Can you work these out from the drawing? Everything is in mm from the part's minimum corner. A direction names the side the tool comes from. Round coordinates to 2 decimals unless told otherwise and drop trailing zeros. Order: outer loops, then holes, each group sorted by start corner. A loop starts at its lowest first (then second) coordinate and runs counter-clockwise, first axis right, second up. Notation, with made-up numbers: M -2,78 L 54,78 A25 ccw 54,100 Z; hole C 1,81.5 d9. An arc over 180 degrees is marked long. Answer as a JSON object with one key per item and string values. Group by question number.
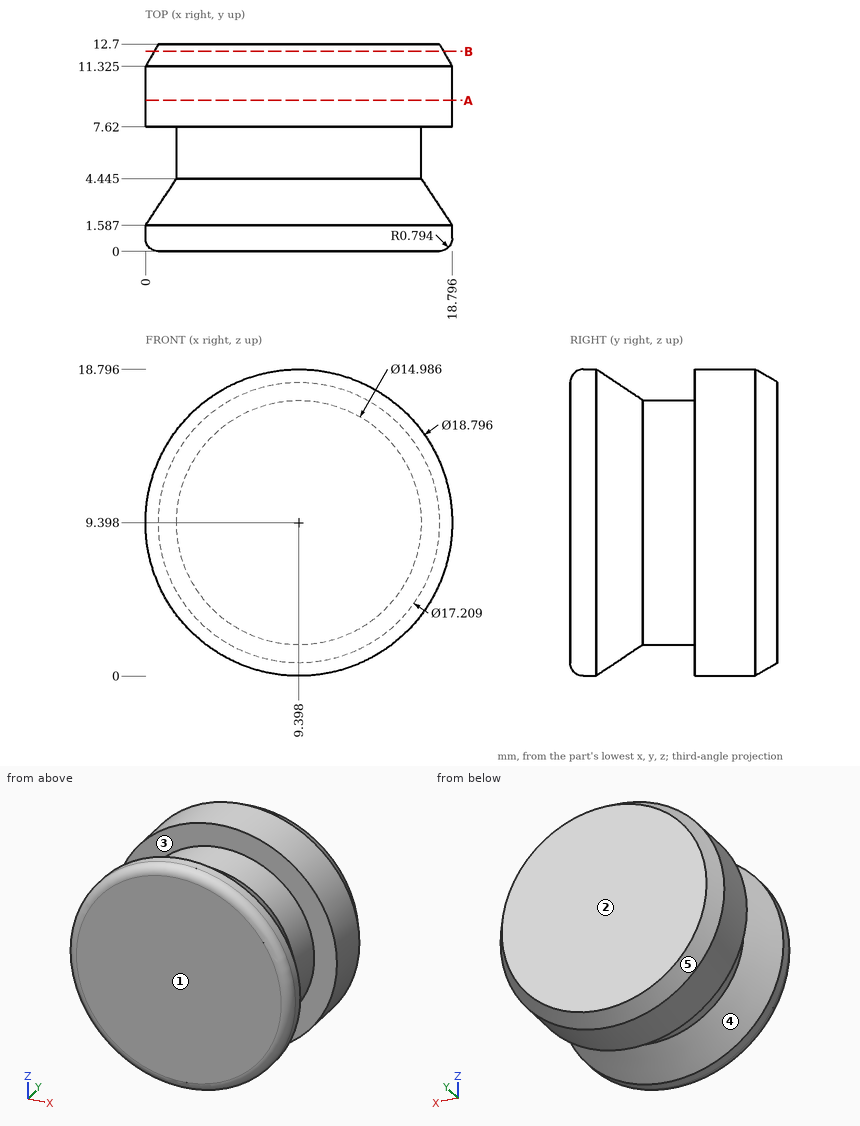
Item 1: On a 3-axis mill with a long thin cutter (end or side, diameter ignored), from which of +Z, -Z, +X, -X, +Y, -Y can I reach the whole of each face in a straight line? I mean the marked faces 4 and 5. Say none if no direction works.
Item 2: Suppose I cut it at A-A, the plane y = 9.25. Write out the boundary of the cut face in (x, z) (1 decimal).
Item 3: If we mould it in two halves opening along Y, with no side actions, what happens to the marked faces 1, 2 and 3? For each: +Y half, -Y half, draft (parallel to the pull), parting line (faces both ways), or undercut.
Item 4: Suppose I cut it at B-B, the plane y = 12.25. Write out the boundary of the cut face in (x, z) (1 decimal), and give its area (3 significant figures).
Item 5: I need wall thicknesses on line 1 (Z direction, x = 9.25, y = 1) (1 decimal); line 2 (Y direction, x = 17, z = 12.5) (1 decimal); line 3 (Y direction, x = 17.75, z = 8) (1 decimal). Which ranges of each line are inside material? Lowest first, please.
Item 6: I'm going to push flat-ended pins straight in: pin 1 Ø2 at (y, z) = (8.5, 17) entering from -X; pin 2 Ø6 at (x, y) = (12, 5) entering from +Z; pin 3 Ø2 at (x, z) = (5, 15) entering from -Y; pin 4 Ø3 at (y, z) = (2.5, 16.5) entering from -X. Where does each tip first touch, or does it pass through?
Computed:
{
 "1": {"face 4": "none", "face 5": "+Y"},
 "2": {"outline": "C 9.4,9.4 d18.8"},
 "3": {"face 1": "-Y half", "face 2": "+Y half", "face 3": "undercut"},
 "4": {"outline": "C 9.4,9.4 d17.7", "area": "247 mm^2"},
 "5": {"line 1": "z = 0 to 18.8", "line 2": "y = 0 to 3.4, 7.6 to 12.7", "line 3": "y = 0 to 3, 7.6 to 12.7"},
 "6": {"pin 1": "stops at x = 2.71", "pin 2": "stops at z = 18.73", "pin 3": "stops at y = 0", "pin 4": "stops at x = 2.09"}
}
